Geometry check sheet. Reference: drawing and pictorial views, mm from the part's lowest x, y, z. A direction names the side the tool comes from. Give positions to 0.01 mm unless a question says otherwise; leave off trailing zeros. Loops run counter-clockwise (first coordinate to the right, second up) from the corner with the lowest first, then second, coordinate; pieces in that order, holes last. Notation, with made-up numbers: (88.25, -16.75) - (138.25, -16.75) arc R13 cw to (138.25, -11.75) - close; hole circle Ø11 at (-34.75, 23.25). An arc over 180 degrees is marked (long way). Put each result on its own line as item: value. Start each with the question number.
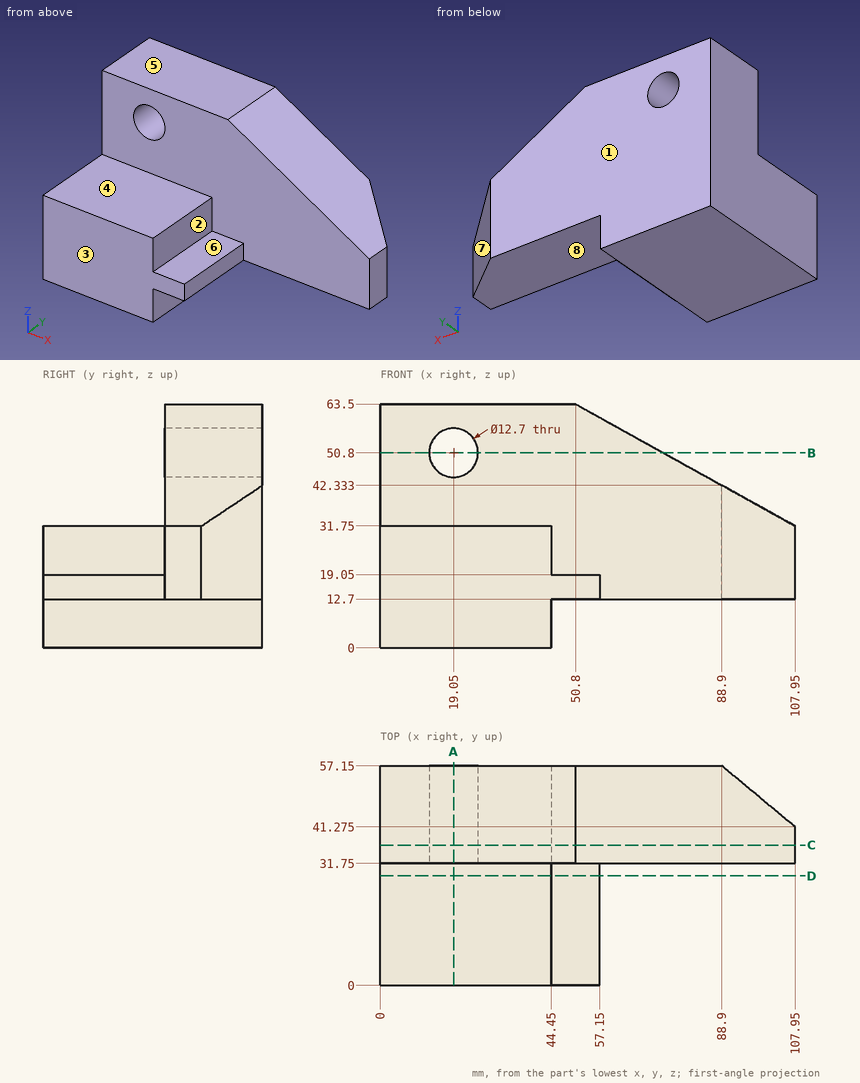
1) Scan lines: line 1 along Z through (x, y) = (19, 46); line 2 along Z through (x, y) = (27, 22); line 3 along Y through (x, z) = (68, 14). Record each from-to range of solid material in increasing order. Write a range as from..to.
2) Section check D-D, the plane y = 28.5. Enter the section's corners in (x, z), plus the area to 3 significant figures.
3) Section check A-A, the plane x = 19.05. Enter the section's corners in (y, z).
4) Section check B-B, the plane z = 50.8. Enter the section's corners in (x, y).
5) Depth check by flat-ended pin: P1, Ø5, axis at y = 23, z = 17, coming from the +X side; P2, Ø14, axis at x = 53.5, y = 17.5, coming from the +Z side; P3, Ø16, axis at x = 17.5, y = 20, coming from the +Z side. Enter the tip coordinate at first touch or a pass-through.
6) Section check C-C, the plane y = 36.5. Enter the section's corners in (x, z), plus the area to 3 significant figures.
7) Set-up check for the marked faces 4, 5, 6, 7 and 8: record each of +Z, -Z, +X, -X, +Y, -Y from which the full face is reachable in a straight line by a thin tool's end or side.
8) Draft check along Y on the marked faces 1, 2 and 3. Enter one of: pulls with the +Y half, pulls with the -Y half, needs draft (parallel to the pull), parting line crosses it, or undercut.
Results are:
1. line 1: z = 0..44.45, 57.15..63.5
1. line 2: z = 0..31.75
1. line 3: y = 31.75..57.15
2. outline: (0, 0) - (44.45, 0) - (44.45, 12.7) - (57.15, 12.7) - (57.15, 19.05) - (44.45, 19.05) - (44.45, 31.75) - (0, 31.75) - close
2. area: 1,490 mm2
3. outline: (0, 0) - (57.15, 0) - (57.15, 44.45) - (31.75, 44.45) - (31.75, 31.75) - (0, 31.75) - close; (31.75, 57.15) - (57.15, 57.15) - (57.15, 63.5) - (31.75, 63.5) - close
4. outline: (0, 31.75) - (12.7, 31.75) - (12.7, 57.15) - (0, 57.15) - close; (25.4, 31.75) - (73.66, 31.75) - (73.66, 57.15) - (25.4, 57.15) - close
5. P1: stops at x = 57.15
5. P2: stops at z = 19.05
5. P3: stops at z = 31.75
6. outline: (0, 0) - (44.45, 0) - (44.45, 12.7) - (107.95, 12.7) - (107.95, 31.75) - (50.8, 63.5) - (0, 63.5) - close; hole circle Ø12.7 at (19.05, 50.8)
6. area: 5,010 mm2
7. face 4: +Z, +X, -X, -Y
7. face 5: +Z, +X, -X, +Y, -Y
7. face 6: +Z, +X, -Y
7. face 7: +Z, -Z, +X, +Y
7. face 8: -Z, +X, +Y, -Y
8. face 1: pulls with the +Y half
8. face 2: needs draft
8. face 3: pulls with the -Y half
